Could you check a few things on this model? Use its own coordinates, in mm. A direction names the side the tool comes from. Coordinates: 2 decimals unless noted, no trailing zeros. Loops run counter-clockwise (first coordinate to the right, second up) from the corner with the lowest first, then second, coordinate; pieces in that order, holes last.
Autodesk Inventor part; units mm, degrees
ref_plane "ABDECKSTOEPSEL_XY" through (0, 0, -7.5) normal (0, 0, -1) x (1, 0, 0)
ref_plane "ABDECKSTOEPSEL_YZ" through (0, 0, -7.5) normal (1, 0, 0) x (0, -1, 0)
ref_plane "ABDECKSTOEPSEL_ZX" through (0, 0, -7.5) normal (0, -1, 0) x (0, 0, -1)
sketch "Sketch_1" plane through (0, 0, 0) normal (0, 0, 1) x (1, 0, 0)
  line L0 (-7.5, -1.5) -> (-7.5, -2)
  line L1 (-7.5, -2) -> (7.5, -2)
  line L2 (7.5, -2) -> (7.5, -1.5)
  line L3 (7.5, -1.5) -> (6, 0)
  line L4 (6, 0) -> (-6, 0)
  line L5 (-6, 0) -> (-7.5, -1.5)
extrude "Extrusion1" add sketch "Sketch_1" along normal mid plane 15
sketch "Sketch_2" plane through (0, 0, 0) normal (1, 0, 0) x (0, 0, -1)
  line L0 (-7.5, -1.5) -> (-6, 0)
  line L1 (-6, 0) -> (6, 0)
  line L2 (6, 0) -> (7.5, -1.5)
  line L3 (7.5, -1.5) -> (7.5, 3.5)
  line L4 (7.5, 3.5) -> (-7.5, 3.5)
  line L5 (-7.5, 3.5) -> (-7.5, -1.5)
extrude "Extrusion2" cut sketch "Sketch_2" along normal mid plane 15
sketch "Sketch_3" plane through (0, -2, 0) normal (0, 1, 0) x (1, 0, 0)
  line L0 (-6.625, -6.625) -> (6.625, -6.625)
  line L1 (6.625, -6.625) -> (6.625, 6.625)
  line L2 (6.625, 6.625) -> (-6.625, 6.625)
  line L3 (-6.625, 6.625) -> (-6.625, -6.625)
  line L4 (-5.625, -5.625) -> (5.625, -5.625)
  line L5 (5.625, -5.625) -> (5.625, 5.625)
  line L6 (5.625, 5.625) -> (-5.625, 5.625)
  line L7 (-5.625, 5.625) -> (-5.625, -5.625)
extrude "Extrusion3" add sketch "Sketch_3" against normal blind 9
sketch "Sketch_4" plane through (0, 0, 0) normal (0, 0, 1) x (1, 0, 0)
  line L0 (-7.5, -9.6) -> (7.5, -9.6)
  line L1 (7.5, -9.6) -> (7.5, -2)
  line L2 (7.5, -2) -> (-7.5, -2)
  line L3 (-7.5, -2) -> (-7.5, -9.6)
extrude "Extrusion4" cut sketch "Sketch_4" along normal mid plane 6
sketch "Sketch_6" plane through (0, 0, 1.125) normal (0, 0, 1) x (1, 0, 0)
  line L0 (5.625, -2.5) -> (5.625, -9.6)
  line L1 (5.625, -9.6) -> (6.625, -9.6)
  line L2 (6.625, -9.6) -> (7.505, -8.0758)
  line L3 (7.505, -8.0758) -> (7.505, -3.0081)
  line L4 (7.505, -3.0081) -> (6.625, -2.5)
  line L5 (6.625, -2.5) -> (5.625, -2.5)
extrude "Extrusion5" add sketch "Sketch_6" along normal mid plane 1.25
sketch "Sketch_7" plane through (0, 0, 1.125) normal (0, 0, 1) x (1, 0, 0)
  line L0 (-7.505, -3.0081) -> (-7.505, -8.0758)
  line L1 (-7.505, -8.0758) -> (-6.625, -9.6)
  line L2 (-6.625, -9.6) -> (-5.625, -9.6)
  line L3 (-5.625, -9.6) -> (-5.625, -2.5)
  line L4 (-5.625, -2.5) -> (-6.625, -2.5)
  line L5 (-6.625, -2.5) -> (-7.505, -3.0081)
extrude "Extrusion6" add sketch "Sketch_7" along normal mid plane 1.25
sketch "Sketch_8" plane through (0, 0, -1.125) normal (0, 0, 1) x (1, 0, 0)
  line L0 (5.625, -2.5) -> (5.625, -9.6)
  line L1 (5.625, -9.6) -> (6.625, -9.6)
  line L2 (6.625, -9.6) -> (7.505, -8.0758)
  line L3 (7.505, -8.0758) -> (7.505, -3.0081)
  line L4 (7.505, -3.0081) -> (6.625, -2.5)
  line L5 (6.625, -2.5) -> (5.625, -2.5)
extrude "Extrusion7" add sketch "Sketch_8" along normal mid plane 1.25
sketch "Sketch_9" plane through (0, 0, -1.125) normal (0, 0, 1) x (1, 0, 0)
  line L0 (-7.505, -3.0081) -> (-7.505, -8.0758)
  line L1 (-7.505, -8.0758) -> (-6.625, -9.6)
  line L2 (-6.625, -9.6) -> (-5.625, -9.6)
  line L3 (-5.625, -9.6) -> (-5.625, -2.5)
  line L4 (-5.625, -2.5) -> (-6.625, -2.5)
  line L5 (-6.625, -2.5) -> (-7.505, -3.0081)
extrude "Extrusion8" add sketch "Sketch_9" along normal mid plane 1.25
ref_plane "ABDECKSTOEPSEL_XY" through (0, 0, -7.5) normal (0, 0, -1) x (1, 0, 0)
ref_plane "ABDECKSTOEPSEL_YZ" through (0, 0, -7.5) normal (1, 0, 0) x (0, -1, 0)
ref_plane "ABDECKSTOEPSEL_ZX" through (0, 0, -7.5) normal (0, -1, 0) x (0, 0, -1)
properties part number "SLZ_63_Abdeck_Stoepsel#"
(1) For pin 1 (1.5 mm diameter, centred on x = -2.5, y = -6, fed in from -Z) (3 decimals); pin 2 (0.5 mm diameter, centred on x = 6.5, z = 0, fed in from +Y); pin 3 (0.8 mm diameter, centred on x = 6.5, z = 2.5, fed in from +Y), each with a flat end and sliding along its axis, tell me the tip position at first contact or that it passes through.
Answers:
pin 1: stops at z = -6.625
pin 2: stops at y = -0.25
pin 3: stops at y = -0.1
(2) Which directions (+Z, -Z, +X, -X, +Y, -Y) give clear straight access to the entire face, cutting with the end or side of a thin tool? Please do faces 3 (the face through (7.071, -2.758, 1.116)), 4 (the face through (-6, -9.6, -2)), 5 (the face through (-7.06, -2.75, 1.12)), 6 (the face through (0, -6, 5.625)).
Answers:
face 3: +Z, -Z, +X
face 4: +X, -X
face 5: +Z, -Z, -X
face 6: -Y
(3) Imagine slicing it at A-A, the plane z = 0. Write out the boundary of the cut face in (x, y) (3 decimals), and give its area (4 significant figures).
Answers:
outline: (-7.5, -2) - (7.5, -2) - (7.5, -1.5) - (6, 0) - (-6, 0) - (-7.5, -1.5) - close; (-6.625, -11) - (-5.625, -11) - (-5.625, -9.6) - (-6.625, -9.6) - close; (5.625, -11) - (6.625, -11) - (6.625, -9.6) - (5.625, -9.6) - close
area: 30.55 mm2
(4) I need wall thicknesses on probe 1 along Z at (x, y) = (-6, -3) (3 decimals); probe 2 along Y at (x, z) = (-6.5, 1.5); probe 3 along X at (y, z) = (-7, 1) (3 decimals). Which ranges of each line are inside material? Lowest first, please.
Answers:
probe 1: z = -6.625 to -3, -1.75 to -0.5, 0.5 to 1.75, 3 to 6.625
probe 2: y = -11 to -2.5, -2 to -0.5
probe 3: x = -7.505 to -5.625, 5.625 to 7.505
(5) Imagine slicing it at B-B, the plane y = -7.5. State how many separate pieces and enclosed holes the cut face has, and give its area (3 significant figures).
Answers:
separate pieces: 6
enclosed holes: 0
area: 46.4 mm2
(6) Imagine slicing it at C-C, the plane x = 4.5. Write out the boundary of the cut face in (y, z) (3 decimals).
Answers:
outline: (-11, -6.625) - (-2, -6.625) - (-2, -7.5) - (-1.5, -7.5) - (0, -6) - (0, 6) - (-1.5, 7.5) - (-2, 7.5) - (-2, 6.625) - (-11, 6.625) - (-11, 5.625) - (-2, 5.625) - (-2, -5.625) - (-11, -5.625) - close
(7) We'd pull the mould along Y, two halves only. Please class faces 1 (the face through (6, -6, 3)), 2 (the face through (0, -6, -6.625)): +Y half, -Y half, draft (parallel to the pull), parting line (faces both ways), or undercut.
Answers:
face 1: undercut
face 2: draft
(8) Imagine slicing it at D-D, the plane z = -3.25. Write out the boundary of the cut face in (x, y) (3 decimals).
Answers:
outline: (-7.5, -2) - (-6.625, -2) - (-6.625, -11) - (-5.625, -11) - (-5.625, -2) - (5.625, -2) - (5.625, -11) - (6.625, -11) - (6.625, -2) - (7.5, -2) - (7.5, -1.5) - (6, 0) - (-6, 0) - (-7.5, -1.5) - close
